```python
from build123d import *

# Parameters (mm, degrees)
F0_W     = 127
F0_H     = 50.8
F1_DEPTH = 25.4
F2_W     = 123.053175
F2_H     = 46.431223
F3_DEPTH = 44.45
F4_R     = 5.031907
F5_DEPTH = 156.464
F6_W     = 60.099678
F6_H     = 12.956048
F7_DEPTH = 78.232


with BuildPart() as f1:
    # F0 (on Top) → F1 (new body)
    with BuildSketch(Plane.XY):
        with Locations((-0.174111, -15.803309)):
            Rectangle(F0_W, F0_H)
    extrude(amount=F1_DEPTH)

    # F2 (on face) → F3 (cut)
    with BuildSketch(Plane.XY.offset(25.4)):
        with Locations((-0.281648, -15.825602)):
            Rectangle(F2_W, F2_H)
    extrude(amount=-F3_DEPTH, mode=Mode.SUBTRACT)

    # F4 (on face) → F5 (cut)
    with BuildSketch(Plane(origin=(-63.674111, 0, 0), x_dir=(0, -1, 0), z_dir=(-1, 0, 0))):
        with Locations((13.734436, 17.974596)):
            Circle(F4_R)
    extrude(amount=-F5_DEPTH, mode=Mode.SUBTRACT)

    # F6 (on face) → F7 (cut)
    with BuildSketch(Plane.XZ.offset(41.203309)):
        with Locations((0.460886, 18.921976)):
            Rectangle(F6_W, F6_H)
    extrude(amount=-F7_DEPTH, mode=Mode.SUBTRACT)


solid = f1.part
```
Design review of the part built by this model. Coordinates are the model's own, in mm. A direction names the side the tool comes from. Give positions to 0.01 mm unless a question says otherwise; leave off trailing zeros. Write each loop counter-clockwise with the first axis right and the second up, starting at its lowest first coordinate (ties: lowest second). Pieces come first, ordered by that corner, then holes.
(1) Add section B-B (y = -26). Give the boundary of the cut face in (x, z), and give its area (3 significant figures).
Checked values:
outline: (-63.67, 0) - (-61.81, 0) - (-61.81, 25.4) - (-63.67, 25.4) - close; (61.24, 0) - (63.33, 0) - (63.33, 25.4) - (61.24, 25.4) - close
area: 100 mm2
(2) Clearance check with flat-ended pins moving along their axes: pin 1 Ø2.5 at (x, y) = (-0.5, -40.5) entering from +Z; pin 2 Ø7.5 at (x, z) = (26.5, 14) entering from -Y; pin 3 Ø6 at (y, z) = (-13.73, 17.97) entering from -X. State where each tip first meets the part, or that it passes through.
Checked values:
pin 1: stops at z = 12.44
pin 2: stops at y = -41.2
pin 3: passes through
(3) Wall thickness on line 1 along X through (y, z) = (6, 17.75); line 2 along Y through (x, z) = (-38, 12.25): over which ranges is each line inside the solid? List them lowest first.
Checked values:
line 1: x = -63.67 to -61.81, 61.24 to 63.33
line 2: y = -41.2 to -39.04, 7.39 to 9.6
(4) Mouldability with a two-part tool opening along X and no side actions: class faces 4 (the face through (63.326, -16, 13)), 5 (the face through (-61.808, -16, 13)), 6 (the face through (0, -40, 0)), 7 (the face through (-29.589, 8, 19)) as +X half, -X half, draft (parallel to the pull), parting line (faces both ways), or undercut.
Checked values:
face 4: +X half
face 5: undercut
face 6: draft
face 7: undercut
(5) Add section C-C (z = 2). Give the boundary of the cut face in (x, y), and give its area (3 significant figures).
Checked values:
outline: (-63.67, -41.2) - (63.33, -41.2) - (63.33, 9.6) - (-63.67, 9.6) - close; hole (-61.81, -39.04) - (61.24, -39.04) - (61.24, 7.39) - (-61.81, 7.39) - close
area: 738 mm2
(6) Tool access review of faces 1 (the face through (-1, -39.041, 10)), 2 (the face through (30.511, -40, 19)), 3 (the face through (-62, -16, 25.4)): name each direction out of +Z, -Z, +X, -X, +Y, -Y from which nothing blocks a thin tool from reaching the whole face with its end or side.
Checked values:
face 1: +Z, -Z
face 2: +Z, +Y, -Y
face 3: +Z, +X, -X, +Y, -Y
(7) Add section D-D (y = -14.5). Give the boundary of the cut face in (x, z).
Checked values:
outline: (-63.67, 0) - (-61.81, 0) - (-61.81, 13) - (-63.67, 13) - close; (-63.67, 22.95) - (-61.81, 22.95) - (-61.81, 25.4) - (-63.67, 25.4) - close; (61.24, 0) - (63.33, 0) - (63.33, 13) - (61.24, 13) - close; (61.24, 22.95) - (63.33, 22.95) - (63.33, 25.4) - (61.24, 25.4) - close
(8) Add section A-A (x = 25.5). Give the boundary of the cut face in (y, z).
Checked values:
outline: (-41.2, 0) - (-39.04, 0) - (-39.04, 12.44) - (-41.2, 12.44) - close; (7.39, 0) - (9.6, 0) - (9.6, 12.44) - (7.39, 12.44) - close
